For this review, use the dimensioned drawing (mm, ordinates from the lowest corner) and the shaded views. A direction names the side the tool comes from. Round coordinates to 2 decimals unless told otherwise and drop trailing zeros. Loops run counter-clockwise (first coordinate to the right, second up) from the corner with the lowest first, then second, coordinate; pieces in that order, holes last. Notation, with made-up numbers: M 62,78 L 118,78 A27 ccw 118,98 Z; hole C 2,-40 d4. An arc over 180 degrees is marked long. One line per item, written item: value. Start each with the question number.
Item 1: We need section A-A (x = 64.5). Write out the cut boundary in (y, z).
Item 2: For line 1 along X through (y, z) = (8.5, 39.5); line 2 along Z through (x, y) = (67.5, 25.5); line 3 along Y through (x, z) = (20, 45), list the stretches that pass through material, from the lowest coordinate up.
Item 3: We need section D-D (y = 17). Write out the cut boundary in (x, z), then the cut area to 3 significant figures.
Item 4: We need section C-C (z = 24). Write out the cut boundary in (x, y), then the cut area to 3 significant figures.
Item 5: We need section B-B (y = 11). Write out the cut boundary in (x, z).
Item 6: Mouldability with a two-part tool opening along X and no side actions: class the marked faces 4, 5, 6 and 7 as released by +X, released by -X, zero draft, split by the parting line, or undercut.
Item 7: For the marked faces 1, 2 and 3, list the 3-axis set-ups (+Z, -Z, +X, -X, +Y, -Y) from which the entire face can be reached by the end or side of a thin tool; tool diameter is ignored.
Item 8: Clearance check with flat-ended pins moving along their axes: pin 1 (6 mm diameter, centred on x = 42, y = 6, fed in from +Z); pin 2 (12 mm diameter, centred on x = 40.5, y = 24, fed in from +Z); pin 3 (4 mm diameter, centred on x = 63, z = 35, fed in from +Y); pin 4 (3 mm diameter, centred on x = 42, z = 40.5, fed in from +Y). State where each tip first meets the part, or that it passes through.
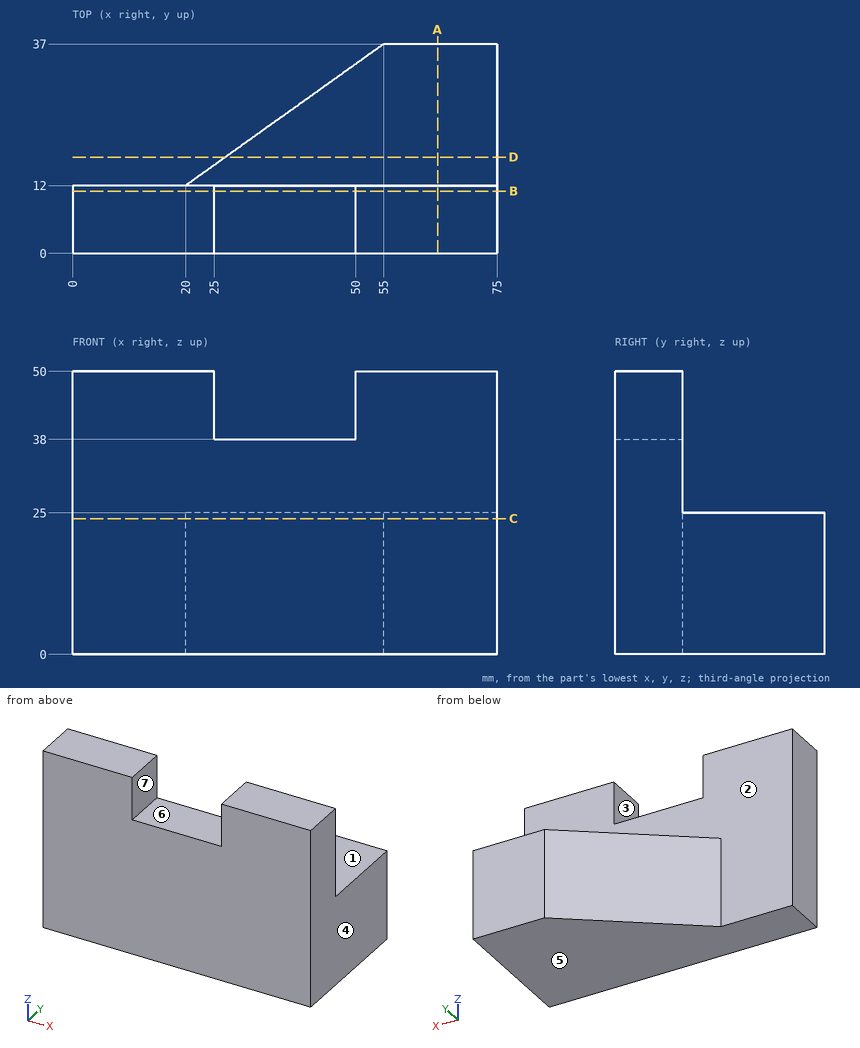
A:
1. outline: M 0,0 L 37,0 L 37,25 L 12,25 L 12,50 L 0,50 Z
2. line 1: 0 to 25, 50 to 75
2. line 2: 0 to 25
2. line 3: 0 to 12
3. outline: M 27,0 L 75,0 L 75,25 L 27,25 Z
3. area: 1,200 mm2
4. outline: M 0,0 L 75,0 L 75,37 L 55,37 L 20,12 L 0,12 Z
4. area: 1,840 mm2
5. outline: M 0,0 L 75,0 L 75,50 L 50,50 L 50,38 L 25,38 L 25,50 L 0,50 Z
6. face 4: released by +X
6. face 5: zero draft
6. face 6: undercut
6. face 7: undercut
7. face 1: +Z, +X, -X, +Y
7. face 2: +Z, -X, +Y
7. face 3: +Z, +Y, -Y
8. pin 1: z = 38
8. pin 2: z = 25
8. pin 3: y = 12
8. pin 4: through
